Drawing for the job (mm, zero at the part's lowest x, y, z). A direction names the side the tool comes from. Coordinates: 2 decimals unless noted, no trailing zeros. Order: outer loops, then holes, each group sorted by start corner. A loop starts at its lowest first (then second) coordinate and runs counter-clockwise, first axis right, second up.
1) Wall check: L1, parallel to X at y = 26, z = 6.5 (1 decimal); L2, parallel to X at y = 22.5, z = 10 (1 decimal); L3, parallel to Y at x = 29, z = 19. Give the ranges that are in metal, low to high.
2) Cut at C-C (y = 21.5). List the corners of the cut face in (x, z), and give its area (3 significant figures).
3) Cut at B-B (y = 12.5). List the corners of the cut face in (x, z) (1 decimal).
4) Cut at A-A (x = 25.5). List the corners of the cut face in (y, z), and give its area (3 significant figures).
5) Cut at D-D (x = 30.5). List the corners of the cut face in (y, z) (1 decimal).
6) Tool access for the marked faces 1 and 2: list every direction of +Z, -Z, +X, -X, +Y, -Y with a clear straight run to the whole face (end or side of a thin tool).
7) Mould opens along Z. For the marked faces 3, 4 and 5 say: +Z half, -Z half, draft (parallel to the pull), parting line (faces both ways), or undercut.
8) Pin check, flat tips, straight feed: pin 1 Ø3 at (y, z) = (29, 8) entering from -X; pin 2 Ø6 at (y, z) = (13.5, 8) entering from +X; pin 3 Ø7 at (y, z) = (22.98, 17.03) entering from -X; pin 4 Ø21.5 at (x, y) = (22.98, 22.98) entering from -Z. Stop position of each tip, or through.
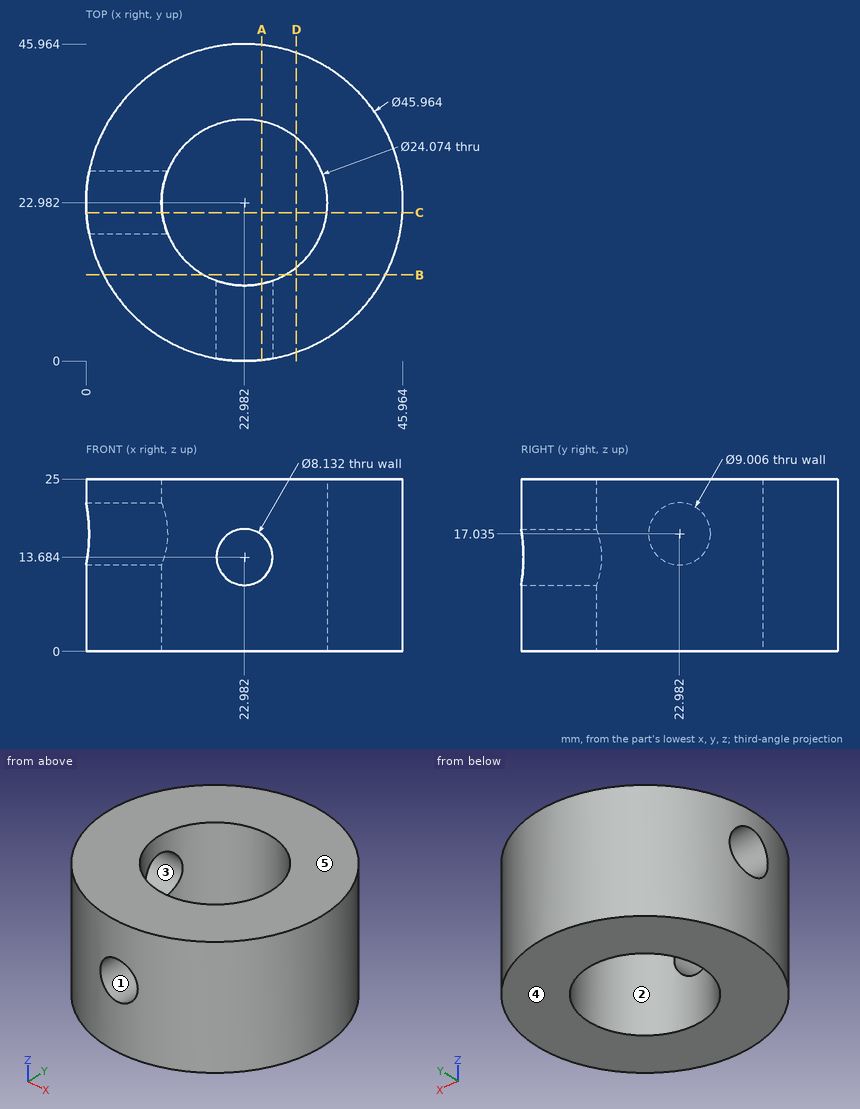
Geometry check:
1. L1: x = 0.2 to 11.3, 34.6 to 45.8
1. L2: x = 0 to 11, 35 to 46
1. L3: y = 0.8 to 12.56, 33.41 to 45.16
2. outline: (0.05, 0) - (11.04, 0) - (11.04, 12.78) - (0.05, 12.78) - close; (0.05, 21.29) - (11.04, 21.29) - (11.04, 25) - (0.05, 25) - close; (34.93, 0) - (45.92, 0) - (45.92, 25) - (34.93, 25) - close
2. area: 456 mm2
3. outline: (2.5, 0) - (17.1, 0) - (17.1, 25) - (2.5, 25) - close; (28.9, 0) - (43.4, 0) - (43.4, 25) - (28.9, 25) - close
4. outline: (0.14, 0) - (11.21, 0) - (11.21, 10.49) - (0.14, 10.49) - close; (0.14, 16.88) - (11.21, 16.88) - (11.21, 25) - (0.14, 25) - close; (34.75, 0) - (45.83, 0) - (45.83, 25) - (34.75, 25) - close
4. area: 483 mm2
5. outline: (1.3, 0) - (13.6, 0) - (13.6, 25) - (1.3, 25) - close; (32.4, 0) - (44.7, 0) - (44.7, 25) - (32.4, 25) - close
6. face 1: -Y
6. face 2: +Z, -Z
7. face 3: undercut
7. face 4: -Z half
7. face 5: +Z half
8. pin 1: stops at x = 0.45
8. pin 2: stops at x = 45.03
8. pin 3: stops at x = 34.5
8. pin 4: passes through
